Input: part model. Units: mm. Frame: model coordinates. A direction names the side the tool comes from. Coordinates: 2 decimals unless noted, no trailing zeros. Write each loop counter-clockwise with the first axis right and the second up, starting at its lowest first coordinate (ties: lowest second). Pieces come first, ordered by that corner, then holes. Notation, with made-up numbers: (23, 33.5) - (32, 33.5) arc R16 ccw to (32, 49.5) - close; hole circle Ø4 at (66.25, 51). An arc over 180 degrees is marked (long way). Use a Markdown table: item, result. Add a question column.
Q1. Section query B-B (z = 88.9). Give the number of separate pieces and of enclosed holes in the cut face, then the cut area to 3 significant figures.
Q2. Section query A-A (x = 5.5). Return the cut outline in (y, z), then the cut area to 3 significant figures.
Q3. Set-up query: faces 4 (the face through (7.802, 6, 64)), 5 (the face through (-12.858, 13.329, 108.037)). Return all of +Z, -Z, +X, -X, +Y, -Y with unobstructed straight access to the full face (end or side cutting, diameter ignored); none if empty.
Q4. Pin query (flat end, axial travel): P1, Ø6, axis at y = 19.01, z = 12.7, coming from the -X side. Return the tip coordinate at first contact, or that it passes through.
Q5. Mould query, pull axis Z, two halves, no side actions, for faces 1 (the face through (-6, 28.534, 64)), 2 (the face through (-0.545, 30.099, 61.235)), 3 (the face through (9.367, -7.569, 61.235)). Classes: released by +Z, released by -Z, zero draft, split by the parting line, or undercut.
Q6. Section query D-D (z = 114.3). Return the cut outline in (x, y).
Q7. Section query C-C (y = 26.5). Return the cut outline in (x, z), then the cut area to 3 significant figures.
Q8. Material intervals for probe 1 along X at (y, z) = (5, 39.5); probe 2 along Y at (x, z) = (-10.5, 111.5); probe 3 along X at (y, z) = (-17, 88.5), sorted ascending. Write a range as from..to.
from build123d import *

# Parameters (mm, degrees)
F0_W     = 25.4
F0_H     = 50.8
F1_DEPTH = 127
F2_W     = 19.05
F2_H     = 44.45
F3_DEPTH = 127
F5_D     = 19.05
F6_D     = 5.1054
F8_D     = 5.1054


# Not quite as in the source:
# - a feature names something its author has since deleted; it is built from what else it names


with BuildPart() as f1:
    # F0 (on Top) → F1 (new body)
    with BuildSketch(Plane.XY):
        with Locations((-1.7230832018, 6.3088932174)):
            Rectangle(F0_W, F0_H)
    extrude(amount=F1_DEPTH)

    # F2 (on face) → F3 (cut)
    with BuildSketch(Plane.XY.offset(127)):
        with Locations((-1.7230832018, 6.3088932174)):
            Rectangle(F2_W, F2_H)
    extrude(amount=-F3_DEPTH, mode=Mode.SUBTRACT)

    # F5 (through all)
    with Locations(Plane.YZ.offset(10.9769167982)):
        with Locations((6.3088932174, 101.6)):
            Hole(F5_D / 2)

    # F6 (through all)
    with Locations(Plane.YZ.offset(10.9769167982)):
        with Locations((-6.3911067826, 63.5), (-6.3911067826, 88.9), (-6.3911067826, 38.1), (-6.3911067826, 12.7), (19.0088932174, 38.1), (19.0088932174, 12.7), (19.0088932174, 63.5), (19.0088932174, 88.9)):
            Hole(F6_D / 2)

    # F8 (through all)
    with Locations(Plane(origin=(0, 31.7088932174, 0), x_dir=(-1, 0, 0), z_dir=(0, 1, 0))):
        with Locations((1.7230832018, 88.9), (1.7230832018, 63.5), (1.7230832018, 114.3), (1.7230832018, 12.7), (1.7230832018, 38.1)):
            Hole(F8_D / 2)


solid = f1.part
Values follow:
| question | item | result |
|---|---|---|
| 1 | separate pieces | 6 |
| 1 | enclosed holes | 0 |
| 1 | area | 346 mm2 |
| 2 | outline | (-19.09, 0) - (-15.92, 0) - (-15.92, 127) - (-19.09, 127) - close; (28.53, 0) - (31.71, 0) - (31.71, 127) - (28.53, 127) - close |
| 2 | area | 806 mm2 |
| 3 | face 4 | +Z, -Z |
| 3 | face 5 | +X, -X |
| 4 | P1 | x = -14.42 |
| 5 | face 1 | zero draft |
| 5 | face 2 | undercut |
| 5 | face 3 | undercut |
| 6 | outline | (-14.42, -19.09) - (-4.28, -19.09) - (-4.28, -15.92) - (-11.25, -15.92) - (-11.25, 28.53) - (-4.28, 28.53) - (-4.28, 31.71) - (-14.42, 31.71) - close; (0.83, -19.09) - (10.98, -19.09) - (10.98, 31.71) - (0.83, 31.71) - (0.83, 28.53) - (7.8, 28.53) - (7.8, -15.92) - (0.83, -15.92) - close |
| 7 | outline | (-14.42, 0) - (-11.25, 0) - (-11.25, 127) - (-14.42, 127) - close; (7.8, 0) - (10.98, 0) - (10.98, 127) - (7.8, 127) - close |
| 7 | area | 806 mm2 |
| 8 | probe 1 | -14.42..-11.25, 7.8..10.98 |
| 8 | probe 2 | -19.09..-15.92, 28.53..31.71 |
| 8 | probe 3 | -14.42..-4.24, 0.8..10.98 |
